Autodesk Inventor part; units mm, degrees
ref_plane "YZ Plane" through (0, 0, 0) normal (1, 0, 0) x (0, 1, 0)
ref_plane "XZ Plane" through (0, 0, 0) normal (0, 1, 0) x (-1, 0, 0)
ref_plane "XY Plane" through (0, 0, 0) normal (0, 0, 1) x (1, 0, 0)
sketch "Эскиз1" plane through (0, 0, 0) normal (0, 0, 1) x (1, 0, 0)
  circle A0 centre (59.533, -59.533) radius 3
  circle A1 centre (-59.533, -59.533) radius 3
  circle A2 centre (-59.533, 59.533) radius 3
  circle A3 centre (59.533, 59.533) radius 3
  circle A4 centre (0, 0) radius 65
  arc A5 (35.5618, 66.033) -> (-35.5618, 66.033) centre (0, 0) ccw
  line L0 (-35.5618, 66.033) -> (-66.033, 66.033)
  line L1 (-66.033, 66.033) -> (-66.033, 35.5618)
  arc A6 (-66.033, 35.5618) -> (-66.033, -35.5618) centre (0, 0) ccw
  line L2 (-66.033, -35.5618) -> (-66.033, -66.033)
  line L3 (-66.033, -66.033) -> (-35.5618, -66.033)
  arc A7 (-35.5618, -66.033) -> (35.5618, -66.033) centre (0, 0) ccw
  line L4 (35.5618, -66.033) -> (66.033, -66.033)
  line L5 (66.033, -66.033) -> (66.033, -35.5618)
  arc A8 (66.033, -35.5618) -> (66.033, 35.5618) centre (0, 0) ccw
  line L6 (66.033, 35.5618) -> (66.033, 66.033)
  line L7 (66.033, 66.033) -> (35.5618, 66.033)
  point P0 (0, 0)
extrude "Выдавливание1" add sketch "Эскиз1" along normal blind 10 contours A4 | L7 L6 A8 L5 L4 A7 L3 L2 A6 L1 L0 A5
sketch "Эскиз8" plane through (0, 0, 0) normal (0, 0, -1) x (-1, 0, 0)
  arc A0 (-18, 26.5) -> (-26.5, 18) centre (-18, 18) ccw
  line L0 (-26.5, -18) -> (-26.5, 18)
  arc A1 (-26.5, -18) -> (-18, -26.5) centre (-18, -18) ccw
  line L1 (18, -26.5) -> (-18, -26.5)
  arc A2 (18, -26.5) -> (26.5, -18) centre (18, -18) ccw
  line L2 (26.5, 18) -> (26.5, -18)
  arc A3 (26.5, 18) -> (18, 26.5) centre (18, 18) ccw
  line L3 (-18, 26.5) -> (18, 26.5)
  circle A4 centre (-21.2132, 21.2132) radius 1.5
  circle A5 centre (-21.2132, -21.2132) radius 1.5
  circle A6 centre (21.2132, -21.2132) radius 1.5
  circle A7 centre (21.2132, 21.2132) radius 1.5
  circle A8 centre (0, 0) radius 22
extrude "Выдавливание6" cut sketch "Эскиз8" against normal blind 10 contours A4 | A5 | A6 | A7
sketch "Эскиз9" plane through (0, 0, 0) normal (0, 0, -1) x (-1, 0, 0)
  line L0 (20.1, -44.6) -> (20.1, 8.5)
  line L1 (20.1, 8.5) -> (15, 14.5)
  line L2 (11.5, 14.5) -> (15, 14.5)
  line L3 (11.5, 14.5) -> (-11.5, 14.5)
  line L4 (-15, 14.5) -> (-11.5, 14.5)
  line L5 (-15, 14.5) -> (-20.1, 8.5)
  line L6 (-20.1, 8.5) -> (-20.1, -44.6)
  line L7 (-20.1, -44.6) -> (-15, -50.6)
  line L8 (-15, -50.6) -> (15, -50.6)
  line L9 (15, -50.6) -> (20.1, -44.6)
  circle A0 centre (11, -47.8) radius 1.025
  circle A1 centre (-11, -47.8) radius 1.025
  circle A2 centre (-17.3, -40) radius 1.025
  circle A3 centre (17.3, -40) radius 1.025
  circle A4 centre (17.3, -18) radius 1.025
  circle A5 centre (17.3, 4) radius 1.025
  circle A6 centre (-17.3, 4) radius 1.025
  circle A7 centre (0, 0) radius 1.55
  circle A8 centre (0, 0) radius 14
  line L10 (-14.5, 11.5) -> (-14.5, -42)
  arc A9 (-11.5, 14.5) -> (-14.5, 11.5) centre (-11.5, 11.5) ccw
  arc A10 (-14.5, -42) -> (-11.5, -45) centre (-11.5, -42) ccw
  line L11 (-20.1, 8.5) -> (-20.1, -44.6)
  arc A11 (14.5, 11.5) -> (11.5, 14.5) centre (11.5, 11.5) ccw
  line L12 (14.5, -42) -> (14.5, 11.5)
  arc A12 (11.5, -45) -> (14.5, -42) centre (11.5, -42) ccw
  line L13 (-11.5, -45) -> (11.5, -45)
  circle A13 centre (-17.3, -18) radius 1.025
extrude "Выдавливание7" cut sketch "Эскиз9" against normal blind 20.75 contours A11 L12 A12 L13 A10 L10 A9 L3 | A0 | A1 | A2 | A3 | A4 | A5 | A6 | A7 | A8 | A13
properties part number "000.202 - Крышка" material "Пластик АБС"
Geometry check sheet. Reference: the model listing, model coordinates, mm. A direction names the side the tool comes from. Give positions to 0.01 mm unless a question says otherwise; leave off trailing zeros. Order: outer loops, then holes, each group sorted by start corner. A loop starts at its lowest first (then second) coordinate and runs counter-clockwise, first axis right, second up.
1. Gauge pin test, flat ends, axial feed: pin 1 Ø3 at (y, z) = (-12.5, 6) entering from +X; pin 2 Ø1 at (y, z) = (25, 3) entering from -X; pin 3 Ø5 at (x, z) = (-1, 2) entering from -Y. Record the tip position at first contact, or that the pin passes through.
2. Section check B-B, the plane y = 49. Enter the section's corners in (x, z).
3. Thickness scan on L1, parallel to Y at x = 60, z = 3.5; L2, parallel to X at y = -1.5, z = 3.5; L3, parallel to Y at x = 11, z = 4.75 (3 decimals). Record the ranges inside material, lowest first.
4. Section check C-C, the plane z = 2. Give the number of separate pieces and of enclosed holes in the cut face, and give its area (3 significant figures).
5. Release check for a two-part mould opening along Y. For faces 5 (the face through (60.917, 62.195, 4.93)), 6 (the face through (66.033, 51, 5)), 7 (the face through (-75, -0.5, 4.9)) record: pulls with the +Y half, pulls with the -Y half, needs draft (parallel to the pull), parting line crosses it, or undercut.
6. Access from +Z, -Z, +X, -X, +Y, -Y to the whole of each face (thin tool, end or side, straight path). Record for faces 1 (the face through (66.033, -51, 5)), 2 (the face through (51, 66.033, 5)), 3 (the face through (14.5, -15, 5)), 4 (the face through (-51, -66.033, 5)).
7. Section check A-A, the plane x = 7. Enter the section's corners in (y, z), and give its area (3 significant figures).
Values follow:
1. pin 1: stops at x = 74.19
1. pin 2: stops at x = -70.89
1. pin 3: stops at y = -75
2. outline: (-66.03, 0) - (66.03, 0) - (66.03, 10) - (-66.03, 10) - close
3. L1: y = -66.03 to -62.5, -56.57 to 56.57, 62.5 to 66.03
3. L2: x = -74.98 to -14.5, 14.5 to 74.98
3. L3: y = -74.189 to -48.825, -46.775 to -45, 14.5 to 74.189
4. separate pieces: 1
4. enclosed holes: 17
4. area: 17,300 mm2
5. face 5: undercut
5. face 6: needs draft
5. face 7: parting line crosses it
6. face 1: +Z, -Z, +X, -Y
6. face 2: +Z, -Z, +X, +Y
6. face 3: +Z, -Z
6. face 4: +Z, -Z, -X, -Y
7. outline: (-74.67, 0) - (-45, 0) - (-45, 10) - (-74.67, 10) - close; (14.5, 0) - (74.67, 0) - (74.67, 10) - (14.5, 10) - close
7. area: 898 mm2
